Work out the finished part from the listing and answer in its coordinate system (mm). A direction names the side the tool comes from. Round coordinates to 2 decimals unless told otherwise and drop trailing zeros. Write each loop counter-clockwise with the first axis right and the second up, starting at its lowest first coordinate (ties: lowest second). Pieces come first, ordered by that corner, then holes.
from build123d import *

# Parameters (mm, degrees)
SKETCH_1_W          = 40
SKETCH_1_H          = 103
EXTRUDE_1_DEPTH     = 5
SKETCH_2_W          = 16
SKETCH_2_H          = 5
CUT_EXTRUDE_2_DEPTH = 5
SKETCH_3_W          = 16
SKETCH_3_H          = 5
EXTRUDE_3_DEPTH     = 5
SKETCH_4_R          = 1
CUT_EXTRUDE_3_DEPTH = 10


with BuildPart() as part:
    # 스케치1 → 보스-돌출1 (new body)
    with BuildSketch(Plane(origin=(0, 0, 0), x_dir=(1, 0, 0), z_dir=(0, 1, 0))):
        with Locations((20, 51.5)):
            Rectangle(SKETCH_1_W, SKETCH_1_H)
    extrude(amount=EXTRUDE_1_DEPTH)

    # 스케치2 → 컷-돌출2 (cut)
    with BuildSketch(Plane(origin=(0, 5, 0), x_dir=(1, 0, 0), z_dir=(0, 1, 0))):
        with Locations((20, 100.5)):
            Rectangle(SKETCH_2_W, SKETCH_2_H)
    extrude(amount=-CUT_EXTRUDE_2_DEPTH, mode=Mode.SUBTRACT)

    # 스케치3 → 보스-돌출3 (add)
    with BuildSketch(Plane(origin=(0, 5, 0), x_dir=(1, 0, 0), z_dir=(0, 1, 0))):
        with Locations((20, -2.5)):
            Rectangle(SKETCH_3_W, SKETCH_3_H)
    extrude(amount=-EXTRUDE_3_DEPTH)

    # 스케치4 → 컷-돌출3 (cut)
    with BuildSketch(Plane(origin=(0, 5, 0), x_dir=(1, 0, 0), z_dir=(0, 1, 0))):
        with Locations((28, -1)):
            Circle(SKETCH_4_R)
        with Locations((12, -1)):
            Circle(SKETCH_4_R)
        with Locations((12, 99)):
            Circle(SKETCH_4_R)
        with Locations((28, 99)):
            Circle(SKETCH_4_R)
    extrude(amount=-CUT_EXTRUDE_3_DEPTH, mode=Mode.SUBTRACT)


solid = part.part
Q1. Find section C-C (x = 31). Determine the outline of the cut face in (y, z).
Q2. A tool of negligible diameter and unlimited length cuts with its end or side. For faces 5 (the face through (6, 2, 0)), 6 (the face through (28, 3, 4)), 7 (the face through (28, 3, -101)), 8 (the face through (29, 3, -99)), from which of +Z, -Z, +X, -X, +Y, -Y can it reach the whole face along a straight path? Write none if from no direction.
Q3. Find section A-A (y = 3.2). Determine the outline of the cut face in (x, z).
Q4. The mould has two halves that part along Z. Classify faces 1 (the face through (6, 2, -103)), 2 (the face through (12, 3, 4)), 3 (the face through (11, 3, -99)), 4 (the face through (27, 3, 1)): +Z half, -Z half, draft (parallel to the pull), parting line (faces both ways), or undercut.
Q5. Given pin 1 (1.5 mm diameter, centred on y = 2, z = 4, fed in from +X); pin 2 (0.9 mm diameter, centred on y = 2, z = 4, fed in from -X); pin 3 (1.5 mm diameter, centred on x = 6.5, y = 3, fed in from +Z), each flat-ended and moving along its own axis, determine where each tip first touches the part or whether it passes through.
Q6. Find section B-B (z = 1). Determine the outline of the cut face in (x, y).
Q7. Find the intervals of material crossed by L1, parallel to Z at x = 10, y = 2.6; L2, parallel to Z at x = 11.5, y = 4.65; L3, parallel to Z at x = 20.5, y = 3.4, in increasing order.
Report:
1. outline: (0, -103) - (5, -103) - (5, 0) - (0, 0) - close
2. face 5: +Z, -X, +Y, -Y
2. face 6: +Z, +X, +Y, -Y
2. face 7: -Z, +Y, -Y
2. face 8: +Y, -Y
3. outline: (0, -103) - (12, -103) - (12, -100) arc R1 cw to (12, -98) - (28, -98) arc R1 cw to (28, -100) - (28, -103) - (40, -103) - (40, 0) - (28, 0) arc R1 cw to (28, 2) - (28, 5) - (12, 5) - (12, 2) arc R1 cw to (12, 0) - (0, 0) - close
4. face 1: -Z half
4. face 2: draft
4. face 3: undercut
4. face 4: undercut
5. pin 1: stops at x = 28
5. pin 2: stops at x = 12
5. pin 3: stops at z = 0
6. outline: (13, 0) - (27, 0) - (27, 5) - (13, 5) - close
7. L1: z = -103 to 0
7. L2: z = -103 to -99.87, -98.13 to 0
7. L3: z = -98 to 5
